Autodesk Inventor part; units mm, degrees
ref_plane "YZ Plane" through (0, 0, 0) normal (1, 0, 0) x (0, 1, 0)
ref_plane "XZ Plane" through (0, 0, 0) normal (0, 1, 0) x (-1, 0, 0)
ref_plane "XY Plane" through (0, 0, 0) normal (0, 0, 1) x (1, 0, 0)
sketch "Boceto1" plane through (0, 0, 0) normal (0, 0, 1) x (1, 0, 0)
  line L0 (0, 55.4788) -> (0, -87.4245) construction
  line L1 (-101.2305, 0) -> (87.3085, 0) construction
  circle A0 centre (0, 0) radius 23.525
  dimension "d0" = 47.05
extrude "Extrusión1" add sketch "Boceto1" along normal blind 7
sketch "Boceto2" plane through (0, 0, 7) normal (0, 0, 1) x (1, 0, 0)
  circle A0 centre (0, 0) radius 20.525
  dimension "d3" = 41.05
extrude "Extrusión2" cut sketch "Boceto2" against normal blind 5
sketch "Boceto4" plane through (0, 0, 2) normal (0, 0, 1) x (1, 0, 0)
  line L0 (0, 23.5497) -> (0, -28.0756) construction
  line L1 (-25.4254, 0) -> (29.9443, 0) construction
  circle A0 centre (0, 0) radius 3
  circle A1 centre (0, 0) radius 12.5 construction
  circle A2 centre (0, 12.5) radius 3
  circle A3 centre (-11.8882, 3.8627) radius 3
  circle A4 centre (-7.3473, -10.1127) radius 3
  circle A5 centre (7.3473, -10.1127) radius 3
  circle A6 centre (11.8882, 3.8627) radius 3
  dimension "d16" = 25
  dimension "d15" = 6
  dimension "d17" = 6
  dimension "d20" = 360
extrude "Extrusión4" add sketch "Boceto4" along normal blind 30
sketch "Boceto5" plane through (0, 0, 32) normal (0, 0, 1) x (1, 0, 0)
  circle A0 centre (0, 0) radius 2
  circle A1 centre (-11.8882, 3.8627) radius 3
  circle A2 centre (-11.8882, 3.8627) radius 2
  circle A3 centre (-7.3473, -10.1127) radius 2
  circle A4 centre (7.3473, -10.1127) radius 2
  circle A5 centre (11.8882, 3.8627) radius 2
  circle A6 centre (0, 12.5) radius 2
  dimension "d24" = 4
  dimension "d25" = 4
  dimension "d28" = 360
extrude "Extrusión5" cut sketch "Boceto5" against normal blind 40 contours A0 | A2 | A3 | A4 | A5 | A6
sketch "Boceto6" plane through (0, 0, 0) normal (0, 0, -1) x (-1, 0, 0)
  circle A0 centre (0, 0) radius 23.525
  dimension "d32" = 47.05
extrude "Extrusión6" add sketch "Boceto6" along normal blind 7
sketch "Boceto7" plane through (0, 0, -7) normal (0, 0, -1) x (-1, 0, 0)
  circle A0 centre (0, 0) radius 2
  circle A1 centre (0, 0) radius 20.525
  dimension "d35" = 41.05
extrude "Extrusión7" cut sketch "Boceto7" against normal blind 7 contours A0 | A1
properties part number "TAPA CAPSULA"
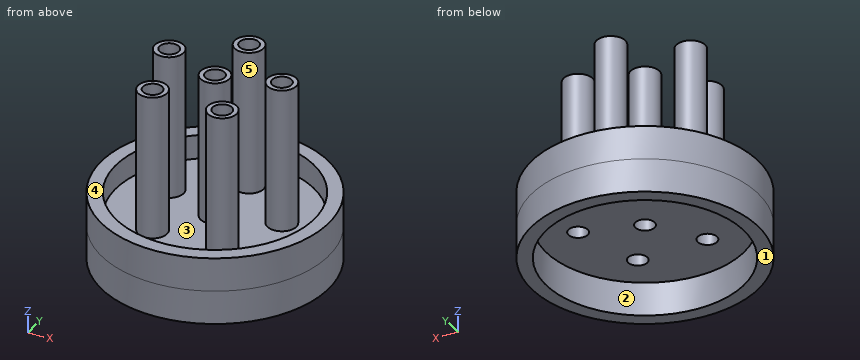
Geometry check sheet. Reference: the model listing, model coordinates, mm. Face numbers are marked on the shaded views. A direction names the side the tool comes from. Coordinates: 2 decimals unless noted, no trailing zeros. Order: outer loops, then holes, each group sorted by start corner. A loop starts at its lowest first (then second) coordinate and runs counter-clockwise, first axis right, second up.
Q1. Sectioned sample at B-B on y = 0. Record the cut outline in (x, z) (3 decimals), and give its area (3 significant figures).
Reply:
outline: (-23.525, -7) - (-20.525, -7) - (-20.525, 0) - (-2, 0) - (-2, 32) - (-3, 32) - (-3, 2) - (-20.525, 2) - (-20.525, 7) - (-23.525, 7) - close; (2, 0) - (20.525, 0) - (20.525, -7) - (23.525, -7) - (23.525, 7) - (20.525, 7) - (20.525, 2) - (3, 2) - (3, 32) - (2, 32) - close
area: 218 mm2
Q2. Depth check by flat-ended pin: pin 1 Ø10 at (x, z) = (6.5, 3) entering from -Y; pin 2 Ø5 at (x, y) = (-11.89, 3.86) entering from -Z; pin 3 Ø1.5 at (x, z) = (7.5, -1.5) entering from -Y; pin 4 Ø23.5 at (x, y) = (-3.5, 11) entering from +Z. Enter the tip coordinate at first touch or a pass-through.
Reply:
pin 1: stops at y = -23.48
pin 2: stops at z = 0
pin 3: stops at y = -22.54
pin 4: stops at z = 32
Q3. Thickness scan on probe 1 along Y at (x, z) = (0, 12.5); probe 2 along Y at (x, z) = (0, -1.75) (3 decimals); probe 3 along X at (y, z) = (0.5, 6). Record the ranges inside material, lowest first.
Reply:
probe 1: y = -3 to -2, 2 to 3, 9.5 to 10.5, 14.5 to 15.5
probe 2: y = -23.525 to -20.525, 20.525 to 23.525
probe 3: x = -23.52 to -20.52, -2.96 to -1.94, 1.94 to 2.96, 20.52 to 23.52
Q4. Sectioned sample at A-A on z = 20. Give the number of separate pieces and of enclosed holes in the cut face, and give its area (3 significant figures).
Reply:
separate pieces: 6
enclosed holes: 6
area: 94.2 mm2
Q5. Sectioned sample at D-D on y = -11. Record the cut outline in (x, z).
Reply:
outline: (-20.79, -7) - (-17.33, -7) - (-17.33, 0) - (-9.14, 0) - (-9.14, 32) - (-10.21, 32) - (-10.21, 2) - (-17.33, 2) - (-17.33, 7) - (-20.79, 7) - close; (-5.55, 0) - (5.55, 0) - (5.55, 32) - (4.48, 32) - (4.48, 2) - (-4.48, 2) - (-4.48, 32) - (-5.55, 32) - close; (9.14, 0) - (17.33, 0) - (17.33, -7) - (20.79, -7) - (20.79, 7) - (17.33, 7) - (17.33, 2) - (10.21, 2) - (10.21, 32) - (9.14, 32) - close
Q6. Sectioned sample at C-C on x = 8. Record the cut outline in (y, z), and give its area (3 significant figures).
Reply:
outline: (-22.12, -7) - (-18.9, -7) - (-18.9, 0) - (-12, 0) - (-12, 32) - (-13.04, 32) - (-13.04, 2) - (-18.9, 2) - (-18.9, 7) - (-22.12, 7) - close; (-8.22, 0) - (18.9, 0) - (18.9, -7) - (22.12, -7) - (22.12, 7) - (18.9, 7) - (18.9, 2) - (-7.18, 2) - (-7.18, 32) - (-8.22, 32) - close
area: 220 mm2
Q7. Tool access check on the marked faces 1, 2 and 3. Record the directions out of +Z, -Z, +X, -X, +Y, -Y that give a thin tool (end or side, any length) a straight path to the whole face; none if there is none.
Reply:
face 1: -Z, +X, -X, +Y, -Y
face 2: -Z
face 3: +Z
Q8. Draft check along Y on the marked faces 4 and 5. Enter one of: released by +Y, released by -Y, zero draft, split by the parting line, or undercut.
Reply:
face 4: zero draft
face 5: undercut
